Geometry check sheet. Reference: the model listing, model coordinates, mm. Face numbers are marked on the shaded views. A direction names the side the tool comes from. Round coordinates to 2 decimals unless told otherwise and drop trailing zeros. Write each loop counter-clockwise with the first axis right and the second up, starting at its lowest first coordinate (ties: lowest second). Pieces come first, ordered by that corner, then holes. Notation, with made-up numbers: (54.5, 47) - (75.5, 47) arc R18 ccw to (75.5, 82) - close; hole circle Ø5 at (35, -2). An arc over 180 degrees is marked (long way). Return JSON: item names as keys, results as strings.
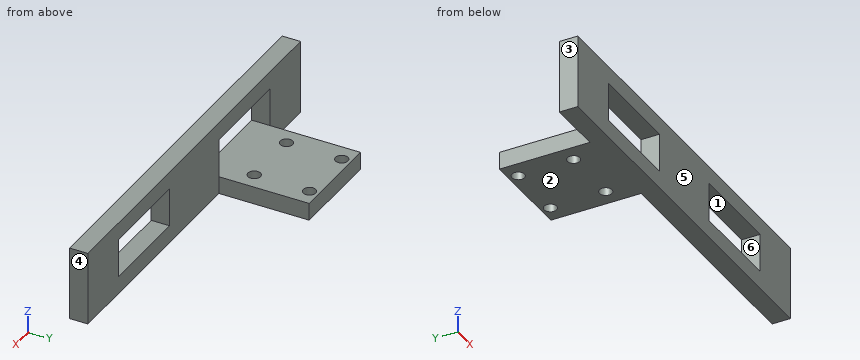
```python
from build123d import *

# Parameters (mm, degrees)
SKETCH1_W           = 105.8
SKETCH1_H           = 20
SKETCH1_W_2         = 25.5
SKETCH1_H_2         = 10.5
BOSS_EXTRUDE1_DEPTH = 5
SKETCH2_W           = 25.5
SKETCH2_H           = 4.75
BOSS_EXTRUDE2_DEPTH = 24.5
SKETCH3_R           = 1.7
CUT_EXTRUDE1_DEPTH  = 5


with BuildPart() as part:
    # Sketch1 → Boss-Extrude1 (new body)
    with BuildSketch(Plane(origin=(0, 0, 0), x_dir=(1, 0, 0), z_dir=(0, 1, 0))):
        Rectangle(SKETCH1_W, SKETCH1_H)
        with Locations((25, 0)):
            Rectangle(SKETCH1_W_2, SKETCH1_H_2, mode=Mode.SUBTRACT)
        with Locations((-25, 0)):
            Rectangle(SKETCH1_W_2, SKETCH1_H_2, mode=Mode.SUBTRACT)
    extrude(amount=BOSS_EXTRUDE1_DEPTH)

    # Sketch2 → Boss-Extrude2 (add)
    with BuildSketch(Plane(origin=(0, 5, 0), x_dir=(1, 0, 0), z_dir=(0, 1, 0))):
        with Locations((-25, 7.625)):
            Rectangle(SKETCH2_W, SKETCH2_H)
    extrude(amount=BOSS_EXTRUDE2_DEPTH)

    # Sketch3 → Cut-Extrude1 (cut)
    with BuildSketch(Plane(origin=(0, 0, -10), x_dir=(-1, 0, 0), z_dir=(0, 0, -1))):
        with Locations((33, 27)):
            Circle(SKETCH3_R)
        with Locations((33, 12)):
            Circle(SKETCH3_R)
        with Locations((17, 12)):
            Circle(SKETCH3_R)
        with Locations((17, 27)):
            Circle(SKETCH3_R)
    extrude(amount=-CUT_EXTRUDE1_DEPTH, mode=Mode.SUBTRACT)


solid = part.part
```
(1) Section check D-D, the plane y = 27. Enter the section's corners in (x, z).
Response values:
{"outline": "(-37.75, -10) - (-34.7, -10) - (-34.7, -5.25) - (-37.75, -5.25) - close; (-31.3, -10) - (-18.7, -10) - (-18.7, -5.25) - (-31.3, -5.25) - close; (-15.3, -10) - (-12.25, -10) - (-12.25, -5.25) - (-15.3, -5.25) - close"}
(2) Section check C-C, the plane y = 3.5. Enter the section's corners in (x, z), plus the area to 3 significant figures.
Response values:
{"outline": "(-52.9, -10) - (52.9, -10) - (52.9, 10) - (-52.9, 10) - close; hole (-37.75, -5.25) - (-12.25, -5.25) - (-12.25, 5.25) - (-37.75, 5.25) - close; hole (12.25, -5.25) - (37.75, -5.25) - (37.75, 5.25) - (12.25, 5.25) - close", "area": "1,580 mm^2"}
(3) Access from +Z, -Z, +X, -X, +Y, -Y to the whole of each face (thin tool, end or side, straight path). Record for the marked faces 5 and 6.
Response values:
{"face 5": "+Z, -Z, +X, -X, -Y", "face 6": "+Y, -Y"}
(4) Release check for a two-part mould opening along X. For the marked faces 1, 2, 3 and 4 record: pulls with the +X half, pulls with the -X half, needs draft (parallel to the pull), parting line crosses it, or undercut.
Response values:
{"face 1": "undercut", "face 2": "needs draft", "face 3": "pulls with the -X half", "face 4": "pulls with the +X half"}
(5) Section check A-A, the plane z = -0.25. Enter the section's corners in (x, y).
Response values:
{"outline": "(-52.9, 0) - (-37.75, 0) - (-37.75, 5) - (-52.9, 5) - close; (-12.25, 0) - (12.25, 0) - (12.25, 5) - (-12.25, 5) - close; (37.75, 0) - (52.9, 0) - (52.9, 5) - (37.75, 5) - close"}
(6) Gauge pin test, flat ends, axial feed: pin 1 (4.5 mm diameter, centred on x = -33, y = 27, fed in from +Z); pin 2 (4 mm diameter, centred on y = 12, z = -7.5, fed in from +X); pin 3 (1.4 mm diameter, centred on y = 22.5, z = -7, fed in from -X). Record the tip position at first contact, or that the pin passes through.
Response values:
{"pin 1": "stops at z = -5.25", "pin 2": "stops at x = -12.25", "pin 3": "stops at x = -37.75"}
(7) Section check B-B, the plane x = -33. Enter the section's corners in (y, z), plus the area to 3 significant figures.
Response values:
{"outline": "(0, -10) - (10.3, -10) - (10.3, -5.25) - (0, -5.25) - close; (0, 5.25) - (5, 5.25) - (5, 10) - (0, 10) - close; (13.7, -10) - (25.3, -10) - (25.3, -5.25) - (13.7, -5.25) - close; (28.7, -10) - (29.5, -10) - (29.5, -5.25) - (28.7, -5.25) - close", "area": "132 mm^2"}
(8) Material ranges on line 1 along Y through (x, z) = (-33, -6.85); line 2 along Y through (x, z) = (-32.5, -7.75); line 3 along X through (y, z) = (21.5, -5.5), recorded low to high. Write a range as [from, to].
Response values:
{"line 1": "y = [0, 10.3], [13.7, 25.3], [28.7, 29.5]", "line 2": "y = [0, 10.38], [13.62, 25.38], [28.62, 29.5]", "line 3": "x = [-37.75, -12.25]"}
